CAD build for the part. Positions are in the model's coordinates, mm. Give positions to 0.01 mm unless a question says otherwise; leave off trailing zeros. Order: outer loops, then holes, each group sorted by start corner. A loop starts at its lowest first (then second) coordinate and runs counter-clockwise, first axis right, second up.
from build123d import *

# Parameters (mm, degrees)
SKETCH1_W           = 120
SKETCH1_H           = 15
SKETCH1_R           = 2.55
BOSS_EXTRUDE1_DEPTH = 2.95
CHAMFER1_SIZE       = 2


with BuildPart() as part:
    # Sketch1 → Boss-Extrude1 (new body)
    with BuildSketch(Plane.XY):
        with Locations((-32.119914347, 29.180942184)):
            Rectangle(SKETCH1_W, SKETCH1_H)
        with Locations((-54.619914347, 29.180942184)):
            Circle(SKETCH1_R, mode=Mode.SUBTRACT)
        with BuildLine():
            Line((0.380085653, 31.680942184), (20.830085653, 31.680942184))
            ThreePointArc((20.830085653, 31.680942184), (23.330085653, 29.180942184), (20.830085653, 26.680942184))
            Line((20.830085653, 26.680942184), (0.380085653, 26.680942184))
            ThreePointArc((0.380085653, 26.680942184), (-2.119914347, 29.180942184), (0.380085653, 31.680942184))
        make_face(mode=Mode.SUBTRACT)
    extrude(amount=BOSS_EXTRUDE1_DEPTH)

    # Chamfer1
    chamfer1_edges = [part.edges().sort_by_distance(p)[0] for p in [
        (27.880085653, 21.680942184, 1.475),
        (-92.119914347, 21.680942184, 1.475),
        (-92.119914347, 36.680942184, 1.475),
        (27.880085653, 36.680942184, 1.475),
    ]]
    chamfer(chamfer1_edges, length=CHAMFER1_SIZE)


solid = part.part
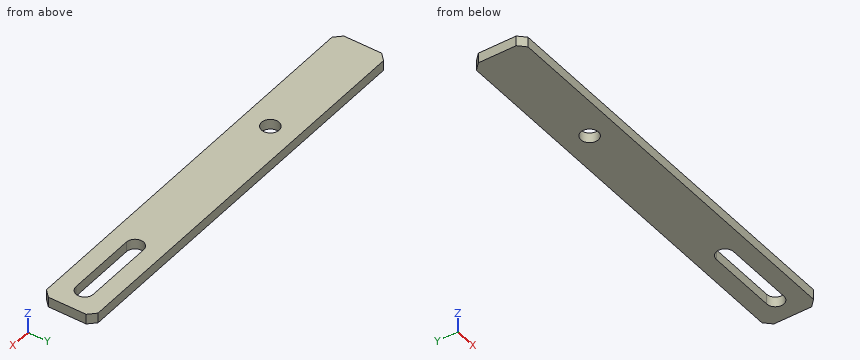
1. Saw through at B-B on y = 30.25. Give the cut face in (x, z) (3 decimals), plus the area to 3 significant figures.
2. Saw through at C-C on z = 2.3. Give the cut face in (x, y).
3. Wall check: line 1 (X direction, y = 29.25, z = 2.15); line 2 (X direction, y = 27.75, z = 2.7); line 3 (Y direction, x = 6, z = 1.75). Give the ranges that are in metal, low to high.
4. Saw through at A-A on x = 5.5. Give the cut face in (y, z).
Reported:
1. outline: (-92.12, 0) - (-56.935, 0) - (-56.935, 2.95) - (-92.12, 2.95) - close; (-52.305, 0) - (-1.88, 0) - (-1.88, 2.95) - (-52.305, 2.95) - close; (23.09, 0) - (27.88, 0) - (27.88, 2.95) - (23.09, 2.95) - close
1. area: 267 mm2
2. outline: (-92.12, 23.68) - (-90.12, 21.68) - (25.88, 21.68) - (27.88, 23.68) - (27.88, 34.68) - (25.88, 36.68) - (-90.12, 36.68) - (-92.12, 34.68) - close; hole circle Ø5.1 at (-54.62, 29.18); hole (0.38, 26.68) - (20.83, 26.68) arc R2.5 ccw to (20.83, 31.68) - (0.38, 31.68) arc R2.5 ccw to start
3. line 1: x = -92.12 to -57.17, -52.07 to -2.12, 23.33 to 27.88
3. line 2: x = -92.12 to -56.73, -52.51 to -1.67, 22.88 to 27.88
3. line 3: y = 21.68 to 26.68, 31.68 to 36.68
4. outline: (21.68, 0) - (26.68, 0) - (26.68, 2.95) - (21.68, 2.95) - close; (31.68, 0) - (36.68, 0) - (36.68, 2.95) - (31.68, 2.95) - close
